from build123d import *

# Parameters (mm, degrees)
BOSS_EXTRUDE1_DEPTH                          = 20
SKETCH2_W                                    = 33
SKETCH2_H                                    = 6
CUT_EXTRUDE1_DEPTH                           = 15
CBORE_FOR_M3_HEX_SOCKET_HEAD_CAP_SCR_2_COUNT = 2
CBORE_FOR_M3_HEX_SOCKET_HEAD_CAP_SCR_2_PITCH = 25
CUT_EXTRUDE2_DEPTH                           = 15
M3_CLEARANCE_HOLE1_D                         = 3.4
M3_CLEARANCE_HOLE1_DEPTH                     = 3


with BuildPart() as part:
    # Sketch1 → Boss-Extrude1 (new body)
    with BuildSketch(Plane(origin=(0, 0, 0), x_dir=(1, 0, 0), z_dir=(0, 1, 0))):
        with BuildLine():
            Line((-31, -1.5), (-16.5, -1.5))
            Line((-16.5, -1.5), (-16.5, -3.5))
            ThreePointArc((-16.5, -3.5), (-12.5, -7.5), (-8.5, -3.5))
            Line((-8.5, -3.5), (-8.5, -1.5))
            Line((-8.5, -1.5), (8.5, -1.5))
            Line((8.5, -1.5), (8.5, -3.5))
            ThreePointArc((8.5, -3.5), (12.5, -7.5), (16.5, -3.5))
            Line((16.5, -3.5), (16.5, -1.5))
            Line((16.5, -1.5), (31, -1.5))
            Line((31, -1.5), (31, 1.5))
            Line((31, 1.5), (-31, 1.5))
            Line((-31, 1.5), (-31, -1.5))
        make_face()
    extrude(amount=BOSS_EXTRUDE1_DEPTH)

    # Sketch2 → Cut-Extrude1 (cut)
    with BuildSketch(Plane(origin=(0, 20, 0), x_dir=(1, 0, 0), z_dir=(0, 1, 0))):
        with Locations((0, -4.5)):
            Rectangle(SKETCH2_W, SKETCH2_H)
    extrude(amount=-CUT_EXTRUDE1_DEPTH, mode=Mode.SUBTRACT)

    # Sketch4 → CBORE for M3 Hex Socket Head Cap Screw1 (revolve, cut)
    with BuildSketch(Plane(origin=(-12.5, 5, 3.5), x_dir=(0, 0, 1), z_dir=(1, 0, 0))):
        Polygon((0, 0), (0, 5), (1.6, 5), (1.6, 3.4), (3.25, 3.4), (3.25, 0), align=None)
    cbore_for_m3_hex_socket_head_cap_screw1 = revolve(axis=Axis((-12.5, 11.35, 3.5), (0, -1, 0)), mode=Mode.SUBTRACT)

    # CBORE for M3 Hex Socket Head Cap Scr 2: CBORE for M3 Hex Socket Head Cap Screw1 ×2
    with Locations(*[(i * CBORE_FOR_M3_HEX_SOCKET_HEAD_CAP_SCR_2_PITCH, 0, 0) for i in range(1, CBORE_FOR_M3_HEX_SOCKET_HEAD_CAP_SCR_2_COUNT)]):
        add(cbore_for_m3_hex_socket_head_cap_screw1, mode=Mode.SUBTRACT)

    # Sketch5 → Cut-Extrude2 (cut)
    with BuildSketch(Plane.XZ.offset(-5)):
        with BuildLine():
            Line((-9.938262309, 1.5), (-15.061737691, 1.5))
            ThreePointArc((-15.061737691, 1.5), (-12.5, 0.25), (-9.938262309, 1.5))
        make_face()
        with BuildLine():
            Line((15.061737691, 1.5), (9.938262309, 1.5))
            ThreePointArc((9.938262309, 1.5), (12.5, 0.25), (15.061737691, 1.5))
        make_face()
    extrude(amount=-CUT_EXTRUDE2_DEPTH, mode=Mode.SUBTRACT)

    # M3 Clearance Hole1
    with Locations(Plane.XY.offset(1.5)):
        with Locations((-28.125, 15), (28.125, 15), (-21, 5), (21, 5), (-27, 7.5), (27, 7.5)):
            Hole(M3_CLEARANCE_HOLE1_D / 2, depth=M3_CLEARANCE_HOLE1_DEPTH)


solid = part.part
Check sheet for the modelled part. Datum: model origin and axes. Units: mm. A direction names the side the tool comes from. Give positions to 0.01 mm unless a question says otherwise; leave off trailing zeros. Write each loop counter-clockwise with the first axis right and the second up, starting at its lowest first coordinate (ties: lowest second). Pieces come first, ordered by that corner, then holes. Notation, with made-up numbers: (17.25, 68) -> (52.25, 68) arc R14 cw to (52.25, 74) -> close; hole circle Ø4 at (88.5, -10.5). An arc over 180 degrees is marked (long way). Use one line per item in the form item = value. Start each with the question number.
1. Section check C-C (z = 5.75). Record the cut outline in (x, y).
2. Mould release check, pull along Z, two halves, no side actions. Record for faces 5 (the flat face through (0, 10, -1.5)), 6 (the cylindrical face through (-13.85, 0.81, 4.36)), 7 (the cylindrical face through (-28.57, 6.85, -0.02)): pulls with the +Z half, pulls with the -Z half, needs draft (parallel to the pull), parting line crosses it, or undercut.
3. Go/stop test with flat-tipped pins: P1, Ø3, axis at x = 11.5, z = 3.5, coming from the +Y side; P2, Ø2, axis at y = 3.5, z = 5, coming from the -X side; P3, Ø8, axis at x = 24.5, y = 6.5, coming from the +Z side. Record where each tip stops, or that it passes through.
4. Section check B-B (x = -21). Record the cut outline in (y, z), and give its area (3 significant figures).
5. Access from +Z, -Z, +X, -X, +Y, -Y to the whole of each face (thin tool, end or side, straight path). Record for faces 1 (the flat face through (-16.5, 2, 2)), 2 (the flat face through (14, 1.6, 2)), 3 (the flat face through (12, 5, 7)), 4 (the flat face through (-8.5, 2, 3)).
6. Thickness scan on line 1 along Z through (x, y) = (-12.5, 2.55); line 2 along Y through (x, z) = (27, 0.3); line 3 along Z through (x, y) = (12.5, 0.45). Record the ranges inside material, lowest first. Write a range as from..to.
7. Section check A-A (y = 15). Record the cut outline in (x, z) (3 decimals).
8. Section check D-D (y = 4). Record the cut outline in (x, z), and give its area (3 significant figures).
Conclusion:
q1.outline = (-15.81, 0) -> (-9.19, 0) -> (-9.19, 5) -> (-10.15, 5) -> (-10.15, 1.6) -> (-14.85, 1.6) -> (-14.85, 5) -> (-15.81, 5) -> close; (9.19, 0) -> (15.81, 0) -> (15.81, 5) -> (14.85, 5) -> (14.85, 1.6) -> (10.15, 1.6) -> (10.15, 5) -> (9.19, 5) -> close
q2.face_5 = pulls with the -Z half
q2.face_6 = undercut
q2.face_7 = needs draft
q3.P1 = 1.6
q3.P2 = -16.47
q3.P3 = 1.5
q4.outline = (0, -1.5) -> (3.3, -1.5) -> (3.3, 1.5) -> (0, 1.5) -> close; (6.7, -1.5) -> (20, -1.5) -> (20, 1.5) -> (6.7, 1.5) -> close
q4.area = 49.8 mm²
q5.face_1 = +Z, -X, +Y, -Y
q5.face_2 = +Y
q5.face_3 = +Z, +X, -X, +Y
q5.face_4 = +Z, +Y, -Y
q6.line_1 = -1.5..0.25, 6.75..7.5
q6.line_2 = 0..5.8, 9.2..13.73, 16.27..20
q6.line_3 = -1.5..1.9, 5.1..7.5
q7.outline = (-31, -1.5) -> (-29.825, -1.5) -> (-29.825, 1.5) -> (-31, 1.5) -> close; (-26.425, -1.5) -> (26.425, -1.5) -> (26.425, 1.5) -> (15.062, 1.5) arc R3.25 cw to (9.938, 1.5) -> (-9.938, 1.5) arc R3.25 cw to (-15.062, 1.5) -> (-26.425, 1.5) -> close; (29.825, -1.5) -> (31, -1.5) -> (31, 1.5) -> (29.825, 1.5) -> close
q8.outline = (-31, -1.5) -> (-22.37, -1.5) -> (-22.37, 1.5) -> (-31, 1.5) -> close; (-19.63, -1.5) -> (19.63, -1.5) -> (19.63, 1.5) -> (16.5, 1.5) -> (16.5, 3.5) arc R4 ccw to (8.5, 3.5) -> (8.5, 1.5) -> (-8.5, 1.5) -> (-8.5, 3.5) arc R4 ccw to (-16.5, 3.5) -> (-16.5, 1.5) -> (-19.63, 1.5) -> close; (22.37, -1.5) -> (31, -1.5) -> (31, 1.5) -> (22.37, 1.5) -> close; hole circle Ø6.5 at (-12.5, 3.5); hole circle Ø6.5 at (12.5, 3.5)
q8.area = 185 mm²
